CAD build for the part. Positions are in the model's coordinates, mm. A direction names the side the tool comes from. Coordinates: 2 decimals unless noted, no trailing zeros. Write each loop counter-clockwise with the first axis right and the second up, starting at its lowest first coordinate (ties: lowest second). Pieces come first, ordered by that corner, then holes. Notation, with made-up numbers: (-35.5, 18) -> (10.5, 18) arc R17 cw to (10.5, 32) -> close; hole circle Ø8 at (-30, -2). An arc over 180 degrees is marked (long way). Answer as CSV lines item,"result".
```python
from build123d import *

# Parameters (mm, degrees)
SKETCH_1_R      = 1.5
EXTRUDE_1_DEPTH = 6


with BuildPart() as part:
    # 草图1 → 凸台-拉伸1 (new body)
    with BuildSketch(Plane(origin=(0, 0, 0), x_dir=(1, 0, 0), z_dir=(0, 1, 0))):
        with BuildLine():
            Line((-9.737949598, 0.947255951), (-9.737949598, -18.902744049))
            ThreePointArc((-9.737949598, -18.902744049), (-4.737949598, -23.902744049), (0.262050402, -18.902744049))
            Line((0.262050402, -18.902744049), (0.262050402, 2.705554152))
            Line((0.262050402, 2.705554152), (-4.737949598, 6.473971492))
            Line((-4.737949598, 6.473971492), (-1.581691427, 9.155643094))
            Line((-1.581691427, 9.155643094), (-2.990655676, 12.582531705))
            ThreePointArc((-2.990655676, 12.582531705), (-4.665394525, 12.928054539), (-6.289924982, 13.461943142))
            Line((-6.289924982, 13.461943142), (-6.197163572, 15.594373686))
            Line((-6.197163572, 15.594373686), (-7.779733646, 14.143748571))
            Line((-7.779733646, 14.143748571), (-7.398920758, 16.220154199))
            ThreePointArc((-7.398920758, 16.220154199), (-7.410512726, 16.226988873), (-7.422097613, 16.233835543))
            Line((-7.422097613, 16.233835543), (-8.875748064, 14.780185092))
            Line((-8.875748064, 14.780185092), (-8.875748064, 17.233009419))
            ThreePointArc((-8.875748064, 17.233009419), (-8.89176269, 17.245719789), (-8.907757306, 17.25845533))
            Line((-8.907757306, 17.25845533), (-10.109322939, 15.658717321))
            Line((-10.109322939, 15.658717321), (-9.864779998, 18.101747371))
            ThreePointArc((-9.864779998, 18.101747371), (-9.900992511, 18.13709659), (-9.937067144, 18.172586506))
            Line((-9.937067144, 18.172586506), (-11.342451387, 16.749598407))
            Line((-11.342451387, 16.749598407), (-10.808718868, 19.12339663))
            ThreePointArc((-10.808718868, 19.12339663), (-10.8603358, 19.186034382), (-10.91156065, 19.248993181))
            Line((-10.91156065, 19.248993181), (-12.466866971, 17.991606109))
            Line((-12.466866971, 17.991606109), (-11.694242841, 20.325491599))
            ThreePointArc((-11.694242841, 20.325491599), (-11.723768007, 20.371016087), (-11.753102902, 20.416663414))
            Line((-11.753102902, 20.416663414), (-13.437877261, 19.338917916))
            Line((-13.437877261, 19.338917916), (-12.397936945, 21.545287297))
            ThreePointArc((-12.397936945, 21.545287297), (-12.412363311, 21.573840278), (-12.426719371, 21.602428674))
            Line((-12.426719371, 21.602428674), (-14.215127033, 20.7071086))
            Line((-14.215127033, 20.7071086), (-12.980819551, 22.874696888))
            ThreePointArc((-12.980819551, 22.874696888), (-12.991659581, 22.903835263), (-13.002429896, 22.932999479))
            Line((-13.002429896, 22.932999479), (-14.879408408, 22.242382606))
            Line((-14.879408408, 22.242382606), (-13.399650606, 24.212499539))
            ThreePointArc((-13.399650606, 24.212499539), (-13.404668281, 24.232259063), (-13.409654964, 24.25202643))
            Line((-13.409654964, 24.25202643), (-15.349283486, 23.764336781))
            Line((-15.349283486, 23.764336781), (-13.663841103, 25.531286293))
            ThreePointArc((-13.663841103, 25.531286293), (-13.666952622, 25.552575019), (-13.670028903, 25.573868865))
            Line((-13.670028903, 25.573868865), (-15.649714954, 25.28953959))
            Line((-15.649714954, 25.28953959), (-13.782119424, 26.702074649))
            Line((-13.782119424, 26.702074649), (-13.786071717, 26.777270326))
            Line((-13.786071717, 26.777270326), (-15.783610509, 26.678079738))
            Line((-15.783610509, 26.678079738), (-13.779118172, 28.19415517))
            ThreePointArc((-13.779118172, 28.19415517), (-13.776521837, 28.236618422), (-13.773786555, 28.27907295))
            Line((-13.773786555, 28.27907295), (-15.769435323, 28.41092892))
            Line((-15.769435323, 28.41092892), (-13.669425272, 29.274347437))
            ThreePointArc((-13.669425272, 29.274347437), (-13.656782501, 29.360141075), (-13.643567704, 29.445848467))
            Line((-13.643567704, 29.445848467), (-15.619182802, 29.757208362))
            Line((-15.619182802, 29.757208362), (-13.388679068, 30.674279319))
            ThreePointArc((-13.388679068, 30.674279319), (-13.368727635, 30.750538102), (-13.348314176, 30.826674507))
            Line((-13.348314176, 30.826674507), (-15.278505654, 31.350469177))
            Line((-15.278505654, 31.350469177), (-12.868620153, 32.341292896))
            Line((-12.868620153, 32.341292896), (-14.692134653, 33.084702139))
            ThreePointArc((-14.692134653, 33.084702139), (-13.851601264, 34.818611239), (-12.795725249, 36.430462034))
            Line((-12.795725249, 36.430462034), (-14.555144967, 40.70972987))
            Line((-14.555144967, 40.70972987), (-18.80498844, 39.992143324))
            ThreePointArc((-18.80498844, 39.992143324), (-22.673158885, 32.282486217), (-21.315703366, 23.764336781))
            Line((-21.315703366, 23.764336781), (-9.737949598, 0.947255951))
        make_face()
        with Locations(Location((-4.737949598, -18.902744049, 0), (0, 0, 270))):
            Circle(SKETCH_1_R, mode=Mode.SUBTRACT)
        with Locations(Location((-4.737949598, 3.097255951, 0), (0, 0, 270))):
            Circle(SKETCH_1_R, mode=Mode.SUBTRACT)
    extrude(amount=EXTRUDE_1_DEPTH)


solid = part.part
```
Item 1: Wall check: line 1 (Z direction, x = -5.25, y = 2.65); line 2 (X direction, y = 1.9, z = 8); line 3 (X direction, y = 1.3, z = -4). Give the ranges that are in metal, low to high. Write a range as from..to.
Answer below:
line 1,"z = -13.1..-4.51, -1.69..17.49, 20.31..23.88"
line 2,"x = -9.74..0.26"
line 3,"x = -11.29..-5.94, -3.54..-1.46"
Item 2: Two-plate mould, pull along X, no slides. Class faces 1 (the flat face through (-2.2, 2.96, -4.56)), 2 (the flat face through (-14.15, 2.958, -23.214)), 3 (the cylindrical face through (-4.85, 2.96, 23.9)): pulls with the +X half, pulls with the -X half, needs draft (parallel to the pull), parting line crosses it, or undercut.
Answer below:
face 1,"pulls with the +X half"
face 2,"undercut"
face 3,"parting line crosses it"
Item 3: 3-axis set-ups, long thin cutter, end or side, ignore diameter. For faces 4 (the flat face through (-6.244, 2.958, -14.513)), 5 (the flat face through (-9.738, 3, 9)), 6 (the cylindrical face through (-4.672, 2.958, 17.404)): which of +Z, -Z, +X, -X, +Y, -Y reach the whole face in a straight line?
Answer below:
face 4,"+X, +Y, -Y"
face 5,"+Z, -X, +Y, -Y"
face 6,"+Y, -Y"
Item 4: Saw through at C-C on z = 3. Give the cut face in (x, y).
Answer below:
outline,"(-9.74, 0) -> (0.26, 0) -> (0.26, 6) -> (-9.74, 6) -> close"
Item 5: Saw through at B-B on y = 5.3. State how many separate pieces and enclosed holes the cut face has, and give its area (3 significant figures).
Answer below:
separate pieces,"1"
enclosed holes,"2"
area,"565 mm2"
Item 6: Saw through at A-A on z = 19.5. Give the cut face in (x, y), and give its area (3 significant figures).
Answer below:
outline,"(-9.7, 0) -> (-6.11, 0) -> (-6.11, 6) -> (-9.7, 6) -> close; (-3.36, 0) -> (0.23, 0) -> (0.23, 6) -> (-3.36, 6) -> close"
area,"43.1 mm2"
Item 7: Flat gauge pins, fed straight in: pin 1 (1.5 mm diameter, centred on y = 4.5, z = -12.5, fed in from -X); pin 2 (2.5 mm diameter, centred on x = -4.74, z = 18.9, fed in from +Y); pin 3 (1.5 mm diameter, centred on x = -17.5, y = 4, fed in from -Z); pin 4 (1.5 mm diameter, centred on y = 3.5, z = -10, fed in from -X). Where does each tip first touch, or does it go through?
Answer below:
pin 1,"stops at x = -15.98"
pin 2,"passes through"
pin 3,"stops at z = -40.34"
pin 4,"stops at x = -14.71"
Item 8: Saw through at D-D on x = -17.25. Give the cut face in (y, z), and give its area (3 significant figures).
Answer below:
outline,"(0, -40.25) -> (6, -40.25) -> (6, -15.75) -> (0, -15.75) -> close"
area,"147 mm2"
